from build123d import *

# Parameters (mm, degrees)
SKETCH056_W     = 150
SKETCH056_H     = 181
PAD017_DEPTH    = 4
SKETCH057_W     = 87
SKETCH057_H     = 17
PAD018_DEPTH    = 13.5
SKETCH058_W     = 155
SKETCH058_H     = 34
PAD019_DEPTH    = 2
SKETCH059_R     = 1.6
POCKET014_DEPTH = 2
SKETCH082_R     = 4.05
POCKET023_DEPTH = 3


with BuildPart() as part:
    # Sketch056 → Pad017 (new body)
    with BuildSketch(Plane.XY):
        with Locations((0, -4)):
            Rectangle(SKETCH056_W, SKETCH056_H)
    extrude(amount=PAD017_DEPTH)

    # Sketch057 (on DatumPlane) → Pad018 (join)
    with BuildSketch(Plane.XY.offset(4)):
        Polygon((-45.5, 86.5), (45.5, 86.5), (45.5, -94.5), (43.5, -94.5), (43.5, 62.5), (-43.5, 62.5), (-43.5, -94.5), (-45.5, -94.5), align=None)
        with Locations((0, 73)):
            Rectangle(SKETCH057_W, SKETCH057_H, mode=Mode.SUBTRACT)
    extrude(amount=PAD018_DEPTH)

    # Sketch058 (on DatumPlane) → Pad019 (join)
    with BuildSketch(Plane.XZ.offset(94.5)):
        with Locations((0, 17)):
            Rectangle(SKETCH058_W, SKETCH058_H)
    extrude(amount=PAD019_DEPTH)

    # Sketch059 (on DatumPlane) → Pocket014 (cut)
    with BuildSketch(Plane.XZ.offset(94.5)):
        with Locations((0, 18)):
            Circle(SKETCH059_R)
    extrude(amount=POCKET014_DEPTH, mode=Mode.SUBTRACT)

    # Sketch082 (on DatumPlane) → Pocket023 (cut)
    with BuildSketch(Plane.XZ.offset(-87)):
        with Locations((0, 8.05)):
            Circle(SKETCH082_R)
    extrude(amount=POCKET023_DEPTH, mode=Mode.SUBTRACT)


with BuildPart() as part_1:
    # Body007 placement: moved
    add(part.part.moved(Location((0, -75.5, -71))))


solid = part_1.part
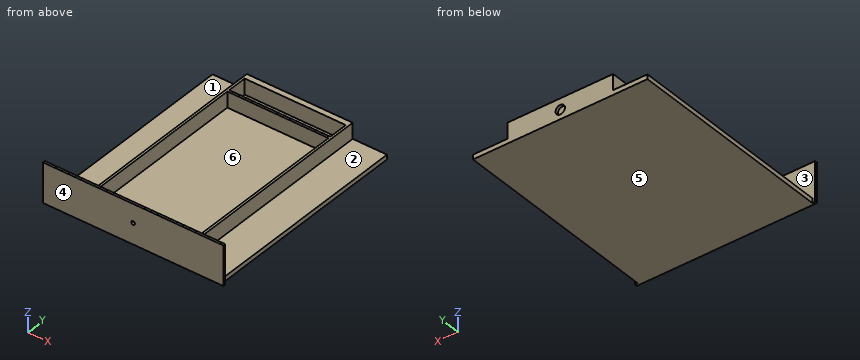
For this review, take the finished solid that the model builds, in its own axes (mm). Face numbers are marked on the shaded views. A direction names the side the tool comes from. Coordinates: 2 decimals unless noted, no trailing zeros. Loops run counter-clockwise (first coordinate to the right, second up) from the corner with the lowest first, then second, coordinate; pieces in that order, holes last. Notation, with made-up numbers: (-32, -26) -> (-26, -26) arc R9 cw to (-26, -20) -> close; hole circle Ø4 at (22.25, -14). An arc over 180 degrees is marked (long way). Write each question's results on one line, items separated by ' | '.
Q1. Add section D-D, the plane z = -40. State the section outline as (x, y) points.
Taken from the geometry:
outline: (-77.5, -172) -> (77.5, -172) -> (77.5, -170) -> (-77.5, -170) -> close
Q2. Machinability: for the marked faces 1, 2, 3 and 4, which of the approach directions +Z, -Z, +X, -X, +Y, -Y give a long, thin tool a straight path to every point of the face, cutting with its end or side? Answer none if there is none.
Taken from the geometry:
face 1: +Z, -X, +Y | face 2: +Z, +X, +Y | face 3: +Z | face 4: +Z, -Z, +X, -X, -Y
Q3. Add section C-C, the plane y = -154. State the section outline as (x, z) points.
Taken from the geometry:
outline: (-75, -71) -> (75, -71) -> (75, -67) -> (45.5, -67) -> (45.5, -53.5) -> (43.5, -53.5) -> (43.5, -67) -> (-43.5, -67) -> (-43.5, -53.5) -> (-45.5, -53.5) -> (-45.5, -67) -> (-75, -67) -> close
Q4. Mouldability with a two-part tool opening along X and no side actions: class the marked faces 5 and 6 as +X half, -X half, draft (parallel to the pull), parting line (faces both ways), or undercut.
Taken from the geometry:
face 5: draft | face 6: undercut
Q5. For pin 1 Ø7 at (y, z) = (0, -61.5) entering from +X; pin 2 Ø18.5 at (x, y) = (-7, -2.5) entering from +Z; pin 3 Ø2 at (y, z) = (-55.5, -54) entering from -X; pin 4 Ø10 at (x, z) = (-8.5, -50.5) entering from +Y, all flat-tipped, find the tip position at first contact; note any pin that passes through.
Taken from the geometry:
pin 1: x = 45.5 | pin 2: z = -53.5 | pin 3: x = -45.5 | pin 4: y = 11
Q6. To check wall thickness, follow line 1 along Y through (x, z) = (22.5, -66); line 2 along X through (y, z) = (-84, -65.5); line 3 along Z through (x, y) = (0, -171.1). State the ranges of each line that lie inside material, in increasing order. Write a range as [from, to].
Taken from the geometry:
line 1: [-172, -170], [-13, -11], [6, 11] | line 2: [-45.5, -43.5], [43.5, 45.5] | line 3: [-71, -54.6], [-51.4, -37]
Q7. Add section A-A, the plane z = -62.95. State the section outline as (x, y) points.
Taken from the geometry:
outline: (-77.5, -172) -> (77.5, -172) -> (77.5, -170) -> (45.5, -170) -> (45.5, 11) -> (4.05, 11) -> (4.05, 8.5) -> (-4.05, 8.5) -> (-4.05, 11) -> (-45.5, 11) -> (-45.5, -170) -> (-77.5, -170) -> close; hole (-43.5, -170) -> (43.5, -170) -> (43.5, -13) -> (-43.5, -13) -> close; hole (-43.5, -11) -> (43.5, -11) -> (43.5, 6) -> (-43.5, 6) -> close
Q8. Add section B-B, the plane x = -36.5. State the section outline as (y, z) points.
Taken from the geometry:
outline: (-172, -71) -> (11, -71) -> (11, -53.5) -> (6, -53.5) -> (6, -67) -> (-11, -67) -> (-11, -53.5) -> (-13, -53.5) -> (-13, -67) -> (-170, -67) -> (-170, -37) -> (-172, -37) -> close
